CAD build for the part. Positions are in the model's coordinates, mm. A direction names the side the tool comes from. Give positions to 0.01 mm unless a question says otherwise; leave off trailing zeros. Write each loop counter-clockwise with the first axis right and the second up, starting at its lowest first coordinate (ties: lowest second). Pieces come first, ordered by that corner, then holes. Notation, with made-up numbers: (33.25, -24.5) - (50.25, -24.5) arc R36 cw to (50.25, 13.5) - close; hole circle Ø9 at (79.5, 4.5). An arc over 180 degrees is marked (long way). Put each result on its own line as item: value. Start each with the question number.
1. Drop flat-ended pins along their axis: pin 1 (1.5 mm diameter, centred on x = -59.5, z = -3, fed in from -Y); pin 2 (4 mm diameter, centred on x = -52.22, z = 4.5, fed in from +Y); pin 3 (4.5 mm diameter, centred on x = -49, z = 11, fed in from -Y); pin 4 (4 mm diameter, centred on x = -102, z = 8, fed in from +Y). Give the stop position or say it passes through.
2. Cut at C-C on x = -111.5. List the corners of the cut face in (y, z), and give its area (3 significant figures).
3. Wall check: line 1 (X direction, y = -1.05, z = 8); line 2 (Z direction, x = -102, y = -2.65); line 3 (X direction, y = -19, z = -3.75). Give the ranges that are in metal, low to high.
4. Tool access for faces 5 (the flat face through (25, 11, 0)), 6 (the flat face through (-51, -5, 7)), 7 (the flat face through (0, -52, -2)), 8 (the flat face through (25, 11, 10)), 9 (the flat face through (20, 11, 5)): list every direction of +Z, -Z, +X, -X, +Y, -Y with a clear straight run to the whole face (end or side of a thin tool).
5. Mould opens along Z. For faces 1 (the cylindrical face through (13.423, -11.778, -2.535)), 2 (the cylindrical face through (-50.604, -2.465, 5.171)), 3 (the flat face through (22, -34, 15)), 4 (the cylindrical face through (5.503, -2.465, 7.846)) say: +Z half, -Z half, draft (parallel to the pull), parting line (faces both ways), or undercut.
6. Cut at D-D on y = 11. List the corners of the cut face in (x, z).
7. Cut at A-A on z = 8. List the corners of the cut face in (x, y).
8. Cut at B-B on y = -78. List the corners of the cut face in (x, z), and give its area (3 significant figures).
from build123d import *

# Parameters (mm, degrees)
BOSS_EXTRUDE3_DEPTH     = 10
SKETCH4_W               = 30
SKETCH4_H               = 25
BOSS_EXTRUDE4_DEPTH     = 5
BOSS_EXTRUDE5_DEPTH     = 5
BOSS_EXTRUDE6_DEPTH     = 71
BOSS_EXTRUDE7_DEPTH     = 124.720470612
SKETCH9_R               = 3.25
CUT_EXTRUDE1_DEPTH      = 15
SKETCH13_R              = 1.75
CUT_EXTRUDE2_DEPTH      = 8
CUT_EXTRUDE2_DEPTH_BACK = 10
SKETCH14_R              = 3.5
CUT_EXTRUDE3_DEPTH      = 8
CUT_EXTRUDE3_DEPTH_BACK = 12
SKETCH15_R              = 3.5
CUT_EXTRUDE4_DEPTH      = 4
CUT_EXTRUDE4_DEPTH_BACK = 17


with BuildPart() as part:
    # Sketch3 → Boss-Extrude3 (new body)
    with BuildSketch(Plane.XY):
        Polygon((0, 0), (0, -5), (20, -5), (20, -25), (30, -25), (30, 22.02), (20, 22.02), (20, 0), align=None)
    extrude(amount=BOSS_EXTRUDE3_DEPTH)

    # Sketch4 → Boss-Extrude4 (add)
    with BuildSketch(Plane(origin=(0, 0, 0), x_dir=(-1, 0, 0), z_dir=(0, 0, -1))):
        with Locations((-15, -12.5)):
            Rectangle(SKETCH4_W, SKETCH4_H)
    extrude(amount=BOSS_EXTRUDE4_DEPTH)

    # Sketch5 → Boss-Extrude5 (add)
    with BuildSketch(Plane.XY.offset(10)):
        Polygon((0, 0), (0, -5), (20, -5), (20, -25), (30, -25), (30, 0), align=None)
    extrude(amount=BOSS_EXTRUDE5_DEPTH)

    # Sketch6 → Boss-Extrude6 (add)
    with BuildSketch(Plane.XZ.offset(25)):
        Polygon((20, 15), (20, 0), (0, 0), (0, -5), (30, -5), (30, 15), align=None)
    extrude(amount=BOSS_EXTRUDE6_DEPTH)

    # Sketch7 → Boss-Extrude7 (add)
    with BuildSketch(Plane.ZY):
        Polygon((15, -5), (15, 0), (0, 0), (-5, 0), (-5, -5), (-5, -9.319004474), (0, -9.319004474), (0, -5), align=None)
    extrude(amount=BOSS_EXTRUDE7_DEPTH)

    # Sketch9 → Cut-Extrude1 (cut)
    with BuildSketch(Plane(origin=(0, 0, -5), x_dir=(-1, 0, 0), z_dir=(0, 0, -1))):
        with Locations((-13, -15)):
            Circle(SKETCH9_R)
    extrude(amount=-CUT_EXTRUDE1_DEPTH, mode=Mode.SUBTRACT)

    # Sketch13 → Cut-Extrude2 (cut, two sides)
    with BuildSketch(Plane(origin=(0, 0, 0), x_dir=(1, 0, 0), z_dir=(0, 1, 0))) as cut_extrude2_sk:
        with Locations((-52.220470612, -4.500931244)):
            Circle(SKETCH13_R)
    extrude(amount=CUT_EXTRUDE2_DEPTH, mode=Mode.SUBTRACT)
    extrude(cut_extrude2_sk.sketch, amount=-CUT_EXTRUDE2_DEPTH_BACK, mode=Mode.SUBTRACT)

    # Sketch14 → Cut-Extrude3 (cut, two sides)
    with BuildSketch(Plane(origin=(0, 0, 0), x_dir=(1, 0, 0), z_dir=(0, 1, 0))) as cut_extrude3_sk:
        with Locations((-102, -8)):
            Circle(SKETCH14_R)
    extrude(amount=CUT_EXTRUDE3_DEPTH, mode=Mode.SUBTRACT)
    extrude(cut_extrude3_sk.sketch, amount=-CUT_EXTRUDE3_DEPTH_BACK, mode=Mode.SUBTRACT)

    # Sketch15 → Cut-Extrude4 (cut, two sides)
    with BuildSketch(Plane(origin=(0, 0, 0), x_dir=(1, 0, 0), z_dir=(0, 1, 0))) as cut_extrude4_sk:
        with Locations((9, -8)):
            Circle(SKETCH15_R)
    extrude(amount=CUT_EXTRUDE4_DEPTH, mode=Mode.SUBTRACT)
    extrude(cut_extrude4_sk.sketch, amount=-CUT_EXTRUDE4_DEPTH_BACK, mode=Mode.SUBTRACT)


solid = part.part
Report:
1. pin 1: stops at y = -9.32
1. pin 2: stops at y = 0
1. pin 3: stops at y = -5
1. pin 4: passes through
2. outline: (-9.32, -5) - (0, -5) - (0, 15) - (-5, 15) - (-5, 0) - (-9.32, 0) - close
2. area: 122 mm²
3. line 1: x = -124.72 to -105.5, -98.5 to 5.5, 12.5 to 30
3. line 2: z = -5 to 4.5, 11.5 to 15
3. line 3: x = 0 to 30
4. face 5: -Z, +X, -X, +Y
4. face 6: +Z, -X, -Y
4. face 7: +Z, -Z, -X, -Y
4. face 8: +Z, +X, -X, +Y
4. face 9: +Z, -Z, -X, +Y
5. face 1: draft
5. face 2: undercut
5. face 3: +Z half
5. face 4: undercut
6. outline: (20, 0) - (30, 0) - (30, 10) - (20, 10) - close
7. outline: (-124.72, -5) - (-105.5, -5) - (-105.5, 0) - (-124.72, 0) - close; (-98.5, -5) - (5.5, -5) - (5.5, 0) - (-98.5, 0) - close; (12.5, -5) - (20, -5) - (20, -96) - (30, -96) - (30, 22.02) - (20, 22.02) - (20, 0) - (12.5, 0) - close
8. outline: (0, -5) - (30, -5) - (30, 15) - (20, 15) - (20, 0) - (0, 0) - close
8. area: 300 mm²
